Could you check a few things on this model? Use its own coordinates, in mm. Round coordinates to 2 decimals unless told otherwise and drop trailing zeros. Loops run counter-clockwise (first coordinate to the right, second up) from the corner with the lowest first, then second, coordinate; pieces in that order, holes last.
from build123d import *

# Parameters (mm, degrees)
SKETCH1_R           = 20
SKETCH1_R_2         = 2.5
BOSS_EXTRUDE1_DEPTH = 10
SKETCH2_R           = 20
BOSS_EXTRUDE2_DEPTH = 15


with BuildPart() as part:
    # Sketch1 → Boss-Extrude1 (new body)
    with BuildSketch(Plane.XY):
        Circle(SKETCH1_R)
        with Locations((0, 15)):
            Circle(SKETCH1_R_2, mode=Mode.SUBTRACT)
        with Locations((10.606601718, 10.606601718)):
            Circle(SKETCH1_R_2, mode=Mode.SUBTRACT)
        with Locations((15, 0)):
            Circle(SKETCH1_R_2, mode=Mode.SUBTRACT)
        with Locations((10.606601718, -10.606601718)):
            Circle(SKETCH1_R_2, mode=Mode.SUBTRACT)
        with Locations((0, -15)):
            Circle(SKETCH1_R_2, mode=Mode.SUBTRACT)
        with Locations((-10.606601718, -10.606601718)):
            Circle(SKETCH1_R_2, mode=Mode.SUBTRACT)
        with Locations((-15, 0)):
            Circle(SKETCH1_R_2, mode=Mode.SUBTRACT)
        with Locations((-10.606601718, 10.606601718)):
            Circle(SKETCH1_R_2, mode=Mode.SUBTRACT)
        with Locations((0, 5)):
            Circle(SKETCH1_R_2, mode=Mode.SUBTRACT)
        with Locations((5, 0)):
            Circle(SKETCH1_R_2, mode=Mode.SUBTRACT)
        with Locations((0, -5)):
            Circle(SKETCH1_R_2, mode=Mode.SUBTRACT)
        with Locations((-5, 0)):
            Circle(SKETCH1_R_2, mode=Mode.SUBTRACT)
    extrude(amount=BOSS_EXTRUDE1_DEPTH)

    # Sketch2 → Boss-Extrude2 (add)
    with BuildSketch(Plane.XY.offset(10)):
        Circle(SKETCH2_R)
    extrude(amount=BOSS_EXTRUDE2_DEPTH)


solid = part.part
Item 1: If we section it at D-D, the plane z = 14.75: Please give me the cut outline in (x, y).
Results list:
outline: circle Ø40 at (0, 0)
Item 2: If I drill on line 1 along Y through (x, z) = (10.5, 2.75); line 2 along X through (y, z) = (9, 9.75); line 3 along Z through (x, y) = (7, -1), over which ranges is the centre line in solid material (lowest first)?
Results list:
line 1: y = -17.02 to -13.1, -8.11 to 8.11, 13.1 to 17.02
line 2: x = -17.86 to -12.52, -8.69 to 8.69, 12.52 to 17.86
line 3: z = 10 to 25
Item 3: Will these pins go through, and if not, where does the flat tip stop? pin 1 (5.5 mm diameter, centred on x = -10, y = -10.5, fed in from -Z); pin 2 (3 mm diameter, centred on y = -6.5, z = 4, fed in from +X); pin 3 (2.5 mm diameter, centred on x = 10.5, y = 11, fed in from -Z); pin 4 (8 mm diameter, centred on x = 2.5, z = 13, fed in from -Y).
Results list:
pin 1: stops at z = 0
pin 2: stops at x = 19.36
pin 3: stops at z = 10
pin 4: stops at y = -20
Item 4: If we section it at B-B, the plane y = 0: Please give me the cut outline in (x, z), then the cut area to 3 significant figures.
Results list:
outline: (-20, 0) - (-17.5, 0) - (-17.5, 10) - (-12.5, 10) - (-12.5, 0) - (-7.5, 0) - (-7.5, 10) - (-2.5, 10) - (-2.5, 0) - (2.5, 0) - (2.5, 10) - (7.5, 10) - (7.5, 0) - (12.5, 0) - (12.5, 10) - (17.5, 10) - (17.5, 0) - (20, 0) - (20, 25) - (-20, 25) - close
area: 800 mm2
Item 5: If we section it at A-A, the plane z = 2.25: Count the separate pieces of the cut face and the enclosed holes in it, then the cut area to 3 significant figures.
Results list:
separate pieces: 1
enclosed holes: 12
area: 1,020 mm2
Item 6: We'd pull the mould along X, two halves only. Please class faces 1 (the flat face through (0, 0, 25)), 2 (the cylindrical face through (-4.336, -19.524, 12.325)), 3 (the cylindrical face through (-12.6, 9.1, 4.9)): released by +X, released by -X, zero draft, split by the parting line, or undercut.
Results list:
face 1: zero draft
face 2: split by the parting line
face 3: undercut
Item 7: If we section it at C-C, the plane x = -5: Please give me the cut outline in (y, z).
Results list:
outline: (-19.36, 0) - (-2.5, 0) - (-2.5, 10) - (2.5, 10) - (2.5, 0) - (19.36, 0) - (19.36, 25) - (-19.36, 25) - close
